from build123d import *

# Parameters (mm, degrees)
BOSS_EXTRUDE1_DEPTH = 38.1
SKETCH2_R           = 1.7272
CUT_EXTRUDE1_DEPTH  = 9.525
SKETCH3_R           = 1.7272
CUT_EXTRUDE2_DEPTH  = 9.525


with BuildPart() as part:
    # Sketch1 → Boss-Extrude1 (new body)
    with BuildSketch(Plane(origin=(0, 0, 0), x_dir=(1, 0, 0), z_dir=(0, 1, 0))):
        Polygon((-2.767735883, 3.334911674), (-1.744793251, 6.855482892), (-4.282226046, 9.501662807), (-7.842601473, 8.627271504), (-8.865544105, 5.106700285), (-6.32811131, 2.46052037), align=None)
    extrude(amount=BOSS_EXTRUDE1_DEPTH)

    # Sketch2 → Cut-Extrude1 (cut)
    with BuildSketch(Plane(origin=(0, 38.1, 0), x_dir=(1, 0, 0), z_dir=(0, 1, 0))):
        with Locations((-5.305168678, 5.981091589)):
            Circle(SKETCH2_R)
    extrude(amount=-CUT_EXTRUDE1_DEPTH, mode=Mode.SUBTRACT)

    # Sketch3 → Cut-Extrude2 (cut)
    with BuildSketch(Plane.XZ):
        with Locations((-5.305168678, -5.981091589)):
            Circle(SKETCH3_R)
    extrude(amount=-CUT_EXTRUDE2_DEPTH, mode=Mode.SUBTRACT)


solid = part.part
Geometry check sheet. Reference: the model listing, model coordinates, mm. A direction names the side the tool comes from. Coordinates: 2 decimals unless noted, no trailing zeros. Loops run counter-clockwise (first coordinate to the right, second up) from the corner with the lowest first, then second, coordinate; pieces in that order, holes last. Notation, with made-up numbers: (-1, 24) - (33, 24) arc R18 cw to (33, 29) - close; hole circle Ø8 at (89, 40). An arc over 180 degrees is marked (long way). Use one line per item in the form item = value. Start each with the question number.
Item 1: Section check A-A, the plane x = -5.25. Enter the section's corners in (y, z) (3 decimals), and give its area (3 significant figures).
Item 2: Tool access check on faces 1 (the face through (-5.7, 33.4, -4.3)), 2 (the face through (-5.53, 4.7, -4.27)), 3 (the face through (-8.347, 18.783, -6.892)). Record the directions out of +Z, -Z, +X, -X, +Y, -Y that give a thin tool (end or side, any length) a straight path to the whole face; none if there is none.
Item 3: Gauge pin test, flat ends, axial feed: pin 1 (1.7 mm diameter, centred on x = -5, z = -5.5, fed in from +Y) (3 decimals); pin 2 (1 mm diameter, centred on x = -8, z = -7.5, fed in from -Y); pin 3 (1.7 mm diameter, centred on x = -5.5, z = -5.5, fed in from -Y) (3 decimals). Record the tip position at first contact, or that the pin passes through.
Item 4: Section check D-D, the plane x = -3.25. Enter the section's corners in (y, z).
Item 5: Thickness scan on probe 1 along X at (y, z) = (2, -7.5); probe 2 along X at (y, z) = (8, -6); probe 3 along Y at (x, z) = (-6, -7) (3 decimals). Record the ranges inside material, lowest first.
Item 6: Section check B-B, the plane y = 18.5. Enter the section's corners in (x, z), and give its area (3 significant figures).
Item 7: Mould release check, pull along X, two halves, no side actions. Record for faces 4 (the face through (-6, 0, -4)), 5 (the face through (-2.263, 18.783, -5.071)), 6 (the face through (-5, 28.575, -6)), 7 (the face through (-6.04, 18.78, -9.07)): +X half, -X half, draft (parallel to the pull), parting line (faces both ways), or undercut.
Item 8: Section check C-C, the plane y = 3. Enter the section's corners in (x, z).
Computed:
q1.outline = (0, -9.264) - (38.1, -9.264) - (38.1, -7.707) - (28.575, -7.707) - (28.575, -4.255) - (38.1, -4.255) - (38.1, -2.725) - (0, -2.725) - (0, -4.255) - (9.525, -4.255) - (9.525, -7.707) - (0, -7.707) - close
q1.area = 183 mm2
q2.face_1 = +Y
q2.face_2 = -Y
q2.face_3 = -Z, -X, +Y, -Y
q3.pin_1 = 28.575
q3.pin_2 = 0
q3.pin_3 = 9.525
q4.outline = (0, -8.43) - (38.1, -8.43) - (38.1, -3.22) - (0, -3.22) - close
q5.probe_1 = -8.17 to -6.13, -4.48 to -2.36
q5.probe_2 = -8.61 to -7.03, -3.58 to -1.99
q5.probe_3 = 9.525 to 28.575
q6.outline = (-8.87, -5.11) - (-7.84, -8.63) - (-4.28, -9.5) - (-1.74, -6.86) - (-2.77, -3.33) - (-6.33, -2.46) - close
q6.area = 34.9 mm2
q7.face_4 = draft
q7.face_5 = +X half
q7.face_6 = undercut
q7.face_7 = -X half
q8.outline = (-8.87, -5.11) - (-7.84, -8.63) - (-4.28, -9.5) - (-1.74, -6.86) - (-2.77, -3.33) - (-6.33, -2.46) - close; hole circle Ø3.45 at (-5.31, -5.98)
